from build123d import *

# Parameters (mm, degrees)
SKETCH_1_W          = 21
SKETCH_1_H          = 19.5
EXTRUDE_1_DEPTH     = 2
SKETCH_3_W          = 15.5
SKETCH_3_H          = 18
EXTRUDE_2_DEPTH     = 13.5
SKETCH_4_W          = 18
SKETCH_4_H          = 4
EXTRUDE_3_DEPTH     = 19.5
SKETCH_2_R          = 7
CUT_EXTRUDE_1_DEPTH = 10
SKETCH_5_R          = 1
CUT_EXTRUDE_2_DEPTH = 10
SKETCH_6_W          = 0.75
SKETCH_6_H          = 3.5
SKETCH_6_W_2        = 3.5
SKETCH_6_H_2        = 0.75
CUT_EXTRUDE_3_DEPTH = 10
SKETCH_7_W          = 1.1
SKETCH_7_H          = 0.3
SKETCH_7_W_2        = 0.8
SKETCH_7_H_2        = 1
SKETCH_7_W_3        = 1
SKETCH_7_H_3        = 0.8
EXTRUDE_4_DEPTH     = 3.5
FILLET_1_R          = 0.5


with BuildPart() as part:
    # Эскиз1 → Бобышка-Вытянуть1 (new body)
    with BuildSketch(Plane.XY):
        with Locations((0, 9.75)):
            Rectangle(SKETCH_1_W, SKETCH_1_H)
    extrude(amount=-EXTRUDE_1_DEPTH)

    # Эскиз3 → Бобышка-Вытянуть2 (add)
    with BuildSketch(Plane.XY):
        with Locations((0, 9)):
            Rectangle(SKETCH_3_W, SKETCH_3_H)
    extrude(amount=-EXTRUDE_2_DEPTH)

    # Эскиз4 → Бобышка-Вытянуть3 (add)
    with BuildSketch(Plane.XY):
        with Locations((0, 2)):
            Rectangle(SKETCH_4_W, SKETCH_4_H)
    extrude(amount=-EXTRUDE_3_DEPTH)

    # Эскиз2 → Вырез-Вытянуть1 (cut)
    with BuildSketch(Plane.XY):
        with Locations((0, 9.75)):
            Circle(SKETCH_2_R)
        with BuildLine():
            Line((-1.25, 15.618347297), (-1.25, 13.25))
            Line((-1.25, 13.25), (1.25, 13.25))
            Line((1.25, 13.25), (1.25, 15.618347297))
            ThreePointArc((1.25, 15.618347297), (0, 3.75), (-1.25, 15.618347297))
        make_face(mode=Mode.SUBTRACT)
    extrude(amount=-CUT_EXTRUDE_1_DEPTH, mode=Mode.SUBTRACT)

    # Эскиз5 → Вырез-Вытянуть2 (cut)
    with BuildSketch(Plane.XY):
        with Locations((0, 6.25)):
            Circle(SKETCH_5_R)
        with Locations((-3, 7.947224362)):
            Circle(SKETCH_5_R)
        with Locations((3, 7.947224362)):
            Circle(SKETCH_5_R)
        with Locations((-3, 11.552775638)):
            Circle(SKETCH_5_R)
        with Locations((3, 11.552775638)):
            Circle(SKETCH_5_R)
        with Locations((0, 9.75)):
            Circle(SKETCH_5_R)
    extrude(amount=-CUT_EXTRUDE_2_DEPTH, mode=Mode.SUBTRACT)

    # Эскиз6 → Вырез-Вытянуть3 (cut)
    with BuildSketch(Plane.XY):
        Polygon((4.516204533, 10.601855654), (1.22728036, 11.798926156), (1.483795467, 12.503695621), (4.77271964, 11.30662512), align=None)
        with Locations((-3, 7.947224362)):
            Rectangle(SKETCH_6_W, SKETCH_6_H)
        with Locations((3, 7.947224362)):
            Rectangle(SKETCH_6_W, SKETCH_6_H)
        with Locations((0, 6.25)):
            Rectangle(SKETCH_6_W, SKETCH_6_H)
        Polygon((-4.516204533, 10.601855654), (-1.22728036, 11.798926156), (-1.483795467, 12.503695621), (-4.77271964, 11.30662512), align=None)
        with Locations((0, 9.75)):
            Rectangle(SKETCH_6_W_2, SKETCH_6_H_2)
    extrude(amount=-CUT_EXTRUDE_3_DEPTH, mode=Mode.SUBTRACT)

    # Эскиз7 → Бобышка-Вытянуть4 (add)
    with BuildSketch(Plane(origin=(0, 0, 0), x_dir=(1, 0, 0), z_dir=(0, 1, 0))):
        with Locations((-5, 3)):
            Rectangle(SKETCH_7_W, SKETCH_7_H)
        with Locations((5, 3)):
            Rectangle(SKETCH_7_W, SKETCH_7_H)
        with Locations((-7.5, 12.4)):
            Rectangle(SKETCH_7_W_2, SKETCH_7_H_2)
        with Locations((0, 12.4)):
            Rectangle(SKETCH_7_W_2, SKETCH_7_H_2)
        with Locations((7.5, 12.4)):
            Rectangle(SKETCH_7_W_2, SKETCH_7_H_2)
        with Locations((-5, 15)):
            Rectangle(SKETCH_7_W_2, SKETCH_7_H_2)
        with Locations((5, 15)):
            Rectangle(SKETCH_7_W_2, SKETCH_7_H_2)
        with Locations((0, 17.3)):
            Rectangle(SKETCH_7_W_3, SKETCH_7_H_3)
    extrude(amount=-EXTRUDE_4_DEPTH)

    # Скругление1
    fillet_1_edges = [part.edges().sort_by_distance(p)[0] for p in [
        (5.55, -3.5, -3),
        (4.45, -3.5, -3),
        (-4.45, -3.5, -3),
        (-5.55, -3.5, -3),
        (0.5, -3.5, -17.3),
        (-0.5, -3.5, -17.3),
        (7.5, -3.5, -12.9),
        (7.5, -3.5, -11.9),
        (5, -3.5, -15.5),
        (5, -3.5, -14.5),
        (0, -3.5, -12.9),
        (0, -3.5, -11.9),
        (-5, -3.5, -14.5),
        (-5, -3.5, -15.5),
        (-7.5, -3.5, -11.9),
        (-7.5, -3.5, -12.9),
    ]]
    fillet(fillet_1_edges, radius=FILLET_1_R - 0.0001)  # a hair under: the kernel refuses the full size


solid = part.part
Part model, mm, in its own coordinate system. A direction names the side the tool comes from. Coordinates: 2 decimals unless noted, no trailing zeros. Write each loop counter-clockwise with the first axis right and the second up, starting at its lowest first coordinate (ties: lowest second). Pieces come first, ordered by that corner, then holes. Notation, with made-up numbers: (-34.75, 33.25) - (-2.75, 33.25) arc R32 cw to (-2.75, 68.25) - close; hole circle Ø2 at (-11, -8). An arc over 180 degrees is marked (long way). Put each result on its own line as item: value.
1. Two-plate mould, pull along X, no slides. Class faces 1 (the cylindrical face through (3.358, 12.487, -4.93)), 2 (the flat face through (9, 2, -11)), 3 (the flat face through (0, 4, -15)): +X half, -X half, draft (parallel to the pull), parting line (faces both ways), or undercut.
Final values:
face 1: undercut
face 2: +X half
face 3: draft
2. Flat gauge pins, fed straight in: pin 1 Ø0.8 at (x, y) = (0, -2.5) entering from +Z; pin 2 Ø1.5 at (y, z) = (1.5, -15.5) entering from -X; pin 3 Ø1 at (x, z) = (0, -3) entering from -Y. Where does each tip first touch, or does it go through?
Final values:
pin 1: stops at z = -11.9
pin 2: stops at x = -9
pin 3: stops at y = 0
3. Band-saw the part on A-A (y = -1.5). Give the number of separate pieces and of enclosed holes in the cut face, then the cut area to 3 significant figures.
Final values:
separate pieces: 8
enclosed holes: 0
area: 5.46 mm²
4. Band-saw the part on D-D (y = 15.25). Write the cut outline in (x, z).
Final values:
outline: (-10.5, -2) - (-7.75, -2) - (-7.75, -13.5) - (7.75, -13.5) - (7.75, -2) - (10.5, -2) - (10.5, 0) - (4.33, 0) - (4.33, -10) - (2.4, -10) - (2.4, 0) - (1.25, 0) - (1.25, -10) - (-1.25, -10) - (-1.25, 0) - (-2.4, 0) - (-2.4, -10) - (-4.33, -10) - (-4.33, 0) - (-10.5, 0) - close
5. 3-axis set-ups, long thin cutter, end or side, ignore diameter. For faces 4 (the flat face through (2.625, 6.6, -4.9)), 5 (the flat face through (7.5, -1.5, -11.9)), 6 (the flat face through (4.6, -2, -15)): which of +Z, -Z, +X, -X, +Y, -Y reach the whole face in a straight line?
Final values:
face 4: +Z
face 5: +Z, +X, -X, -Y
face 6: -Z, -Y
6. Probe line 1 along Y through (x, z) = (-5, -9.25); line 2 along Y through (x, z) = (8.5, -5.75); line 3 along Y through (x, z) = (1.75, -12.25). List the from-to ranges inside material, lowest first. Write a range as [from, to].
Final values:
line 1: y = [0, 4.85], [6.43, 13.07], [14.65, 18]
line 2: y = [0, 4]
line 3: y = [0, 18]
